Answer from the drawing. Dimensions are ordinates in mm from the lowest x, y and z of the part. A direction names the side the tool comes from. Round coordinates to 2 decimals unless told otherwise and drop trailing zeros. Loops run counter-clockwise (first coordinate to the right, second up) from the corner with the lowest first, then second, coordinate; pieces in that order, holes last. Notation, with made-up numbers: M 9,-26.75 L 68,-26.75 A21 ccw 68,11.25 Z; hole C 48,25.25 d10. An arc over 180 degrees is marked long. Answer as a JSON object with one key per item and string values.
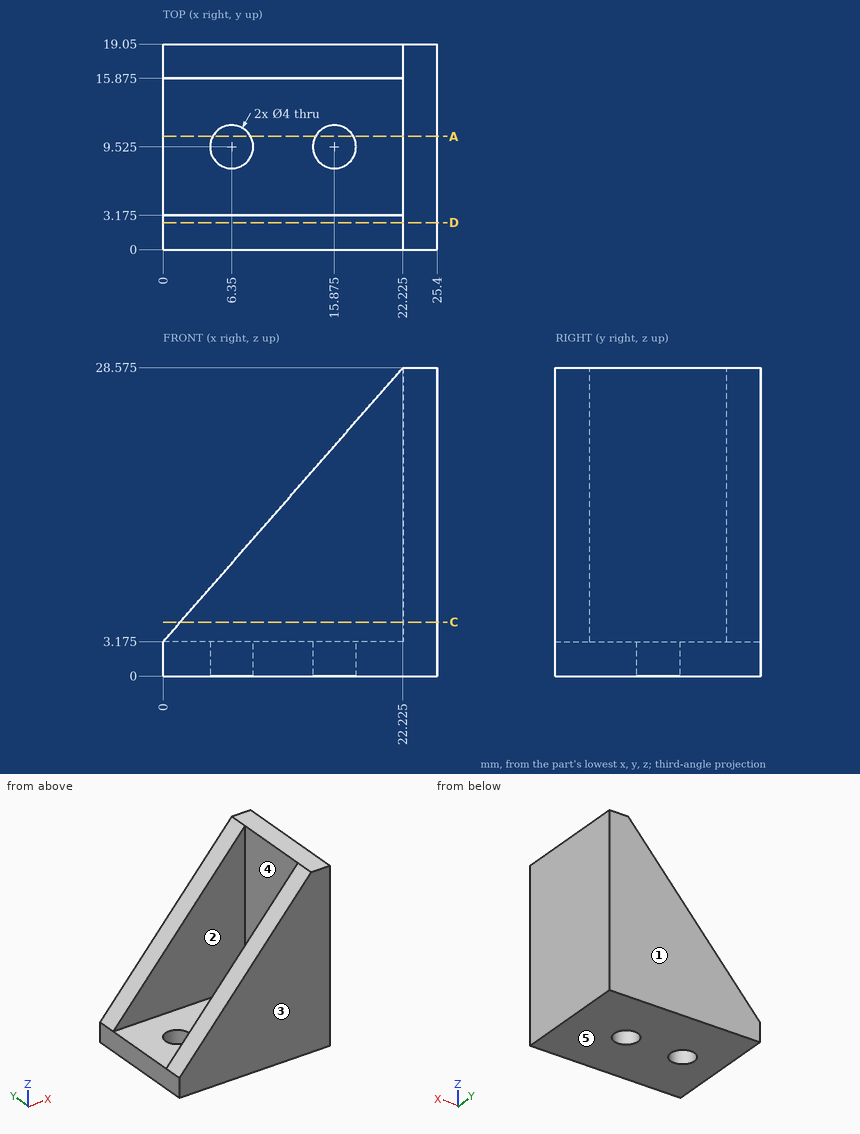
Item 1: Straight lines are drawn through the part: line 1 (Y direction, x = 9, z = 4) (3 decimals); line 2 (Y direction, x = 6.35, z = 0.7) (3 decimals); line 3 (X direction, y = 14, z = 10.5) (3 decimals). For each, find the intervals that lie inside material, in ascending order.
Values follow:
{"line 1": "0 to 3.175, 15.875 to 19.05", "line 2": "0 to 7.525, 11.525 to 19.05", "line 3": "22.225 to 25.4"}
Item 2: The part is cut by section A-A (y = 10.5). Give the vertices of the cut face in (x, z) (3 decimals), then the cut area to 3 significant figures.
Values follow:
{"outline": "M 0,0 L 4.604,0 L 4.604,3.175 L 0,3.175 Z; M 8.096,0 L 14.129,0 L 14.129,3.175 L 8.096,3.175 Z; M 17.621,0 L 25.4,0 L 25.4,28.575 L 22.225,28.575 L 22.225,3.175 L 17.621,3.175 Z", "area": "139 mm^2"}
Item 3: Flat-ended cylindrical pins translate along their axes: P1, Ø3.5, axis at x = 15.875, y = 9.525, coming from the -Z side; P2, Ø4, axis at y = 9, z = 13, coming from the -X side (3 decimals); P3, Ø4, axis at x = 10, y = 7.5, coming from the +Z side (3 decimals). Find the tip coordinate at first contact, or state that the pin passes through.
Values follow:
{"P1": "through", "P2": "x = 22.225", "P3": "z = 3.175"}
Item 4: Which of the six approach directions +Z, -Z, +X, -X, +Y, -Y give full straight-line access (tool end or side, diameter ignored) to the marked faces 4 and 5?
Values follow:
{"face 4": "+Z, -X", "face 5": "-Z, +X, -X, +Y, -Y"}
Item 5: The part is cut by section C-C (z = 5). Give the vertices of the cut face in (x, y) (3 decimals), then the cut area to 3 significant figures.
Values follow:
{"outline": "M 1.597,0 L 25.4,0 L 25.4,19.05 L 1.597,19.05 L 1.597,15.875 L 22.225,15.875 L 22.225,3.175 L 1.597,3.175 Z", "area": "191 mm^2"}
Item 6: The part is cut by section D-D (y = 2.5). Give the vertices of the cut face in (x, z) (3 decimals), then the cut area to 3 significant figures.
Values follow:
{"outline": "M 0,0 L 25.4,0 L 25.4,28.575 L 22.225,28.575 L 0,3.175 Z", "area": "444 mm^2"}
Item 7: Determine the mould class of the marked faces 1, 2 and 3 for opening direction Y: released by +Y, released by -Y, zero draft, split by the parting line, or undercut.
Values follow:
{"face 1": "released by +Y", "face 2": "undercut", "face 3": "released by -Y"}
